Job drawing, mm, ordinate dimensions from the low corner. One solid piece. A direction names the side the tool comes from. Coordinates: 2 decimals unless noted, no trailing zeros. Order: outer loops, then holes, each group sorted by start corner. A loop starts at its lowest first (then second) coordinate and runs counter-clockwise, first axis right, second up. Notation, with made-up numbers: (34.25, 60) - (71.25, 60) arc R21 cw to (71.25, 94) - close; hole circle Ø2 at (35, 78.25). An arc over 180 degrees is marked (long way). Use a Markdown table: item, result. Add a question column.
1) Wall check: L1, parallel to Y at x = 12.7, z = 0.65; L2, parallel to Z at x = 7, y = 5.5. Give the ranges that are in metal, low to high. Write a range as [from, to].
2) Saw through at C-C on y = 6.35. List the corners of the cut face in (x, z).
3) Drop a flat-ended pin along its axis: P1, Ø2, axis at x = 15, y = 6.5, coming from the +Z side. Give the stop position or say it passes through.
4) Saw through at D-D on y = 2.5. List the corners of the cut face in (x, z).
5) Tool access for the marked faces 1 and 2: list every direction of +Z, -Z, +X, -X, +Y, -Y with a clear straight run to the whole face (end or side of a thin tool).
6) Saw through at A-A on x = 12.7. List the corners of the cut face in (y, z).
7) Saw through at B-B on z = 12.7. List the corners of the cut face in (x, y).
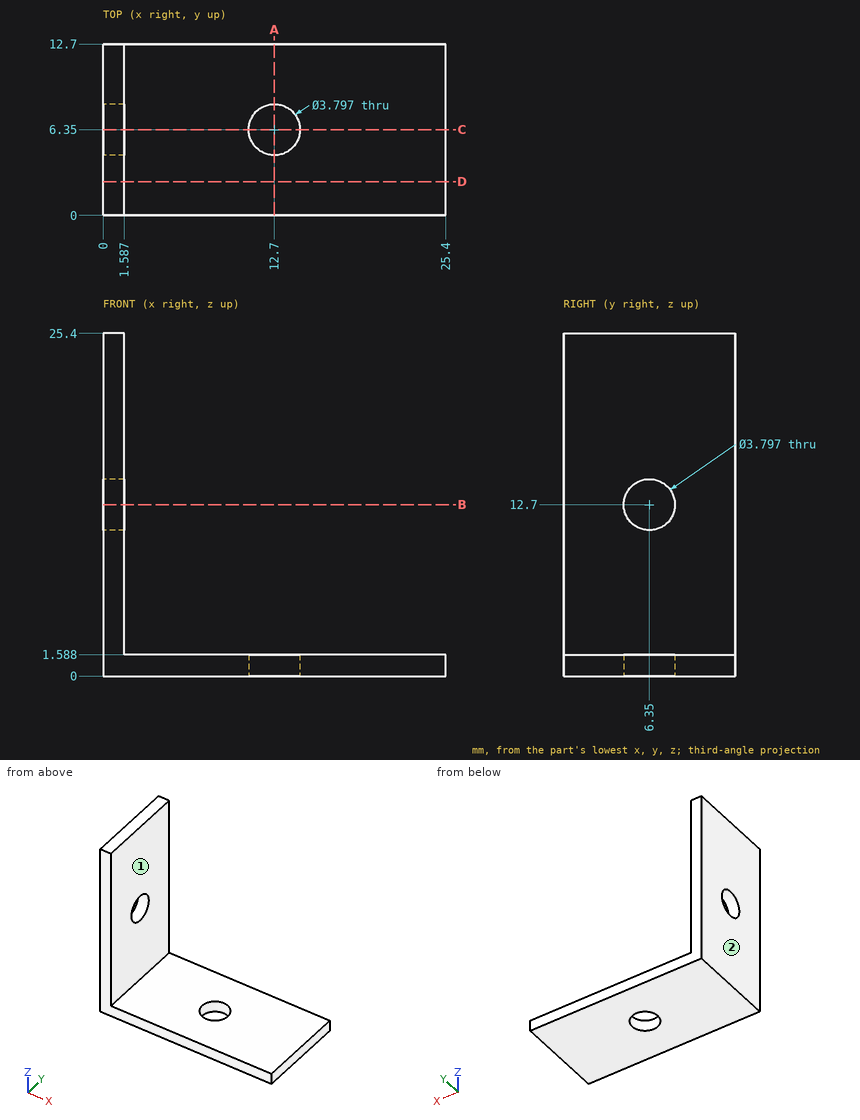
Results are:
| question | item | result |
|---|---|---|
| 1 | L1 | [0, 4.45], [8.25, 12.7] |
| 1 | L2 | [0, 1.59] |
| 2 | outline | (0, 0) - (10.8, 0) - (10.8, 1.59) - (1.59, 1.59) - (1.59, 10.8) - (0, 10.8) - close; (0, 14.6) - (1.59, 14.6) - (1.59, 25.4) - (0, 25.4) - close; (14.6, 0) - (25.4, 0) - (25.4, 1.59) - (14.6, 1.59) - close |
| 3 | P1 | z = 1.59 |
| 4 | outline | (0, 0) - (25.4, 0) - (25.4, 1.59) - (1.59, 1.59) - (1.59, 25.4) - (0, 25.4) - close |
| 5 | face 1 | +Z, +X, +Y, -Y |
| 5 | face 2 | +Z, -Z, -X, +Y, -Y |
| 6 | outline | (0, 0) - (4.45, 0) - (4.45, 1.59) - (0, 1.59) - close; (8.25, 0) - (12.7, 0) - (12.7, 1.59) - (8.25, 1.59) - close |
| 7 | outline | (0, 0) - (1.59, 0) - (1.59, 4.45) - (0, 4.45) - close; (0, 8.25) - (1.59, 8.25) - (1.59, 12.7) - (0, 12.7) - close |
